The drawing under review shows one solid part. Ordinate dimensions are in mm from its lowest x, y, z. A direction names the side the tool comes from. Give positions to 0.01 mm unless a question says otherwise; leave off trailing zeros. Loops run counter-clockwise (first coordinate to the right, second up) from the corner with the lowest first, then second, coordinate; pieces in that order, holes last. Notation, with made-up numbers: M 82,65 L 90,65 A31 ccw 90,101 Z; hole C -21.5,-14.75 d1. An arc over 180 degrees is marked long. Answer as CSV lines item,"result".
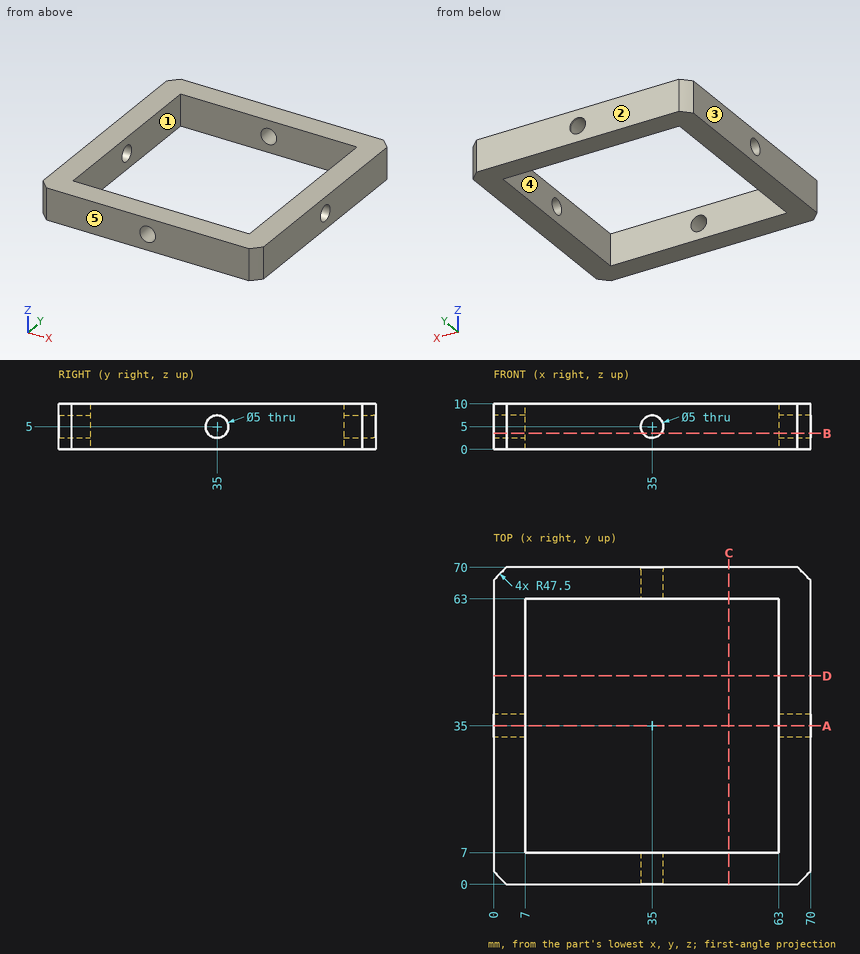
1. We need section C-C, the plane x = 52. Write out the cut boundary in (y, z), plus the area to 3 significant figures.
Answer block:
outline,"M 0,0 L 7,0 L 7,10 L 0,10 Z; M 63,0 L 70,0 L 70,10 L 63,10 Z"
area,"140 mm²"
2. The part is to be moulded in two halves that separate along Y. For the marked faces 3, 4 and 5, say which applies: pulls with the +Y half, pulls with the -Y half, needs draft (parallel to the pull), parting line crosses it, or undercut.
Answer block:
face 3,"needs draft"
face 4,"undercut"
face 5,"pulls with the -Y half"
3. To check wall thickness, follow L1, parallel to X at y = 20, z = 4.5; L2, parallel to Z at x = 35, y = 65. State the ranges of each line that lie inside material, in increasing order. Write a range as [from, to].
Answer block:
L1,"[0, 7], [63, 70]"
L2,"[0, 2.5], [7.5, 10]"
4. We need section B-B, the plane z = 3.5. Write out the cut boundary in (x, y).
Answer block:
outline,"M 0,2.89 A47.5 ccw 2.89,0 L 33,0 L 33,7 L 7,7 L 7,33 L 0,33 Z; M 0,37 L 7,37 L 7,63 L 33,63 L 33,70 L 2.89,70 A47.5 ccw 0,67.11 Z; M 37,0 L 67.11,0 A47.5 ccw 70,2.89 L 70,33 L 63,33 L 63,7 L 37,7 Z; M 37,63 L 63,63 L 63,37 L 70,37 L 70,67.11 A47.5 ccw 67.11,70 L 37,70 Z"
5. We need section A-A, the plane y = 35. Write out the cut boundary in (x, z).
Answer block:
outline,"M 0,0 L 7,0 L 7,2.5 L 0,2.5 Z; M 0,7.5 L 7,7.5 L 7,10 L 0,10 Z; M 63,0 L 70,0 L 70,2.5 L 63,2.5 Z; M 63,7.5 L 70,7.5 L 70,10 L 63,10 Z"
6. For the marked faces 1 and 2, list the 3-axis set-ups (+Z, -Z, +X, -X, +Y, -Y) from which the entire face can be reached by the end or side of a thin tool; tool diameter is ignored.
Answer block:
face 1,"+Z, -Z"
face 2,"+Z, -Z, +X, -X, +Y"
